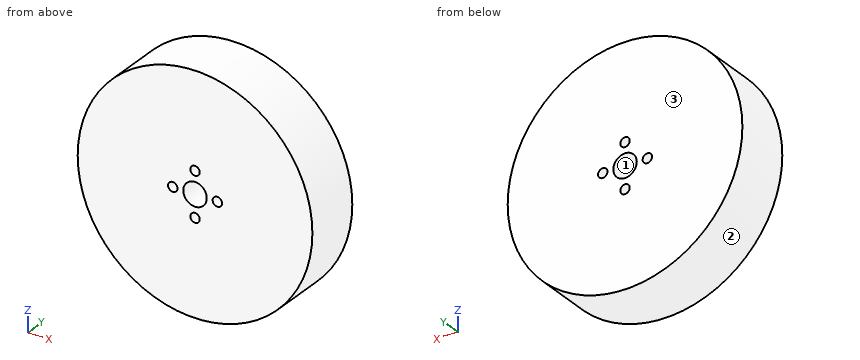
Autodesk Inventor part; units mm, degrees
ref_plane "YZ Plane" through (0, 0, 0) normal (1, 0, 0) x (0, 1, 0)
ref_plane "XZ Plane" through (0, 0, 0) normal (0, 1, 0) x (-1, 0, 0)
ref_plane "XY Plane" through (0, 0, 0) normal (0, 0, 1) x (1, 0, 0)
sketch "Sketch1" plane through (0, 0, 0) normal (0, 1, 0) x (-1, 0, 0)
  circle A0 centre (0, 0) radius 50.8
  circle A1 centre (0, 0) radius 5.08
  dimension "d0" = 101.6
  dimension "d1" = 10.16
extrude "Extrusion1" add sketch "Sketch1" along normal blind 25.4
sketch "Sketch2" plane through (0, 25.4, 0) normal (0, 1, 0) x (1, 0, 0)
  circle A0 centre (0, 0) radius 5.08
  line L0 (-5.08, 0) -> (-9.652, 0)
  circle A1 centre (-9.652, 0) radius 2.032
  dimension "d4" = 4.572
  dimension "d5" = 4.064
extrude "Extrusion2" cut sketch "Sketch2" against normal blind 25.4 contours A1
sketch "Sketch3" plane through (0, 25.4, 0) normal (0, 1, 0) x (1, 0, 0)
  point P0 (0, 0)
  point P1 (0, 0)
pattern_circular "Circular Pattern1" count 4 over 360 about axis through (0, 25.4, 0) along (0, 1, 0) of "Extrusion2"
properties part number "w"
Model file for the job. Use its own axes, mm. Face numbers are marked on the shaded views. Give positions to 0.01 mm unless a question says otherwise; leave off trailing zeros. Order: outer loops, then holes, each group sorted by start corner. A loop starts at its lowest first (then second) coordinate and runs counter-clockwise, first axis right, second up. Notation, with made-up numbers: (17, -20) - (25, -20) arc R23 cw to (25, -3) - close; hole circle Ø2 at (25.5, 7.25). An arc over 180 degrees is marked (long way). One line per item, written item: value.
Item 1: Wall check: line 1 (Z direction, x = -37.5, y = 8.75); line 2 (Z direction, x = -21, y = 16); line 3 (X direction, y = 8, z = -30). Give the ranges that are in metal, low to high.
Response values:
line 1: -34.27 to 34.27
line 2: -46.26 to 46.26
line 3: -41 to 41
Item 2: Slice it at A-A (x = 0). List the corners of the cut face in (y, z).
Response values:
outline: (0, -50.8) - (25.4, -50.8) - (25.4, -11.68) - (0, -11.68) - close; (0, -7.62) - (25.4, -7.62) - (25.4, -5.08) - (0, -5.08) - close; (0, 5.08) - (25.4, 5.08) - (25.4, 7.62) - (0, 7.62) - close; (0, 11.68) - (25.4, 11.68) - (25.4, 50.8) - (0, 50.8) - close
Item 3: Slice it at B-B (z = 0). List the corners of the cut face in (x, y).
Response values:
outline: (-50.8, 0) - (-11.68, 0) - (-11.68, 25.4) - (-50.8, 25.4) - close; (-7.62, 0) - (-5.08, 0) - (-5.08, 25.4) - (-7.62, 25.4) - close; (5.08, 0) - (7.62, 0) - (7.62, 25.4) - (5.08, 25.4) - close; (11.68, 0) - (50.8, 0) - (50.8, 25.4) - (11.68, 25.4) - close
Item 4: Pin check, flat tips, straight feed: pin 1 Ø3.5 at (x, z) = (0, -9.652) entering from -Y; pin 2 Ø8 at (x, y) = (32.5, 17) entering from +Z; pin 3 Ø5.5 at (x, z) = (-9.652, 0) entering from +Y; pin 4 Ø2 at (y, z) = (4, 14.5) entering from -X. Stop position of each tip, or through.
Response values:
pin 1: through
pin 2: z = 42.05
pin 3: y = 25.4
pin 4: x = -48.97
Item 5: Two-plate mould, pull along Z, no slides. Class the marked faces 1, 2 and 3: released by +Z, released by -Z, zero draft, split by the parting line, or undercut.
Response values:
face 1: undercut
face 2: split by the parting line
face 3: zero draft
Item 6: Slice it at D-D (x = 40). List the corners of the cut face in (y, z).
Response values:
outline: (0, -31.32) - (25.4, -31.32) - (25.4, 31.32) - (0, 31.32) - close
Item 7: Slice it at C-C (y = 7.5). List the corners of the cut face in (x, z).
Response values:
outline: circle Ø101.6 at (0, 0); hole circle Ø4.06 at (-9.65, 0); hole circle Ø10.16 at (0, 0); hole circle Ø4.06 at (0, -9.65); hole circle Ø4.06 at (0, 9.65); hole circle Ø4.06 at (9.65, 0)
